Check sheet for the modelled part. Datum: model origin and axes. Units: mm. Round coordinates to 2 decimals unless told otherwise and drop trailing zeros. Write each loop counter-clockwise with the first axis right and the second up, starting at its lowest first coordinate (ties: lowest second). Pieces come first, ordered by that corner, then holes.
Item 1: Cross-section at A-A on y = 0.75. Enter the section's corners in (x, z).
Item 2: Go/stop test with flat-tipped pins: pin 1 Ø1.2 at (x, z) = (-55, -90) entering from -Y; pin 2 Ø3 at (x, z) = (55, 90) entering from +Y. Record where each tip stops, or that it passes through.
Item 3: Material ranges on line 1 (X direction, y = 0.5, z = 90); line 2 (X direction, y = 0.35, z = 68); line 3 (Z direction, x = -62, y = 1.55), recorded low to high.
Item 4: Cross-section at B-B on x = -78. Enter the section's corners in (y, z), plus the area to 3 significant figures.
from build123d import *

# Parameters (mm, degrees)
ESBO_O1_W                = 190
ESBO_O1_H                = 190
RESSALTO_EXTRUS_O1_DEPTH = 1.6
FILETE1_R                = 35
ESBO_O2_R                = 1
CORTE_EXTRUS_O1_DEPTH    = 135.359815421


with BuildPart() as part:
    # Esboço1 → Ressalto-extrusão1 (new body)
    with BuildSketch(Plane(origin=(0, 0, 0), x_dir=(1, 0, 0), z_dir=(0, 1, 0))):
        Rectangle(ESBO_O1_W, ESBO_O1_H)
    extrude(amount=RESSALTO_EXTRUS_O1_DEPTH)

    # Filete1
    filete1_edges = [part.edges().sort_by_distance(p)[0] for p in [
        (95, 0.8, 95),
        (-95, 0.8, 95),
        (-95, 0.8, -95),
        (95, 0.8, -95),
    ]]
    fillet(filete1_edges, radius=FILETE1_R)

    # Esboço2 → Corte-extrusão1 (cut, through all)
    with BuildSketch(Plane(origin=(0, 1.6, 0), x_dir=(1, 0, 0), z_dir=(0, 1, 0))):
        with Locations(Location((-55, 90, 0), (0, 0, 270))):
            Circle(ESBO_O2_R)
        with Locations(Location((55, 90, 0), (0, 0, 90))):
            Circle(ESBO_O2_R)
        with Locations(Location((55, -90, 0), (0, 0, 270))):
            Circle(ESBO_O2_R)
        with Locations(Location((-55, -90, 0), (0, 0, 90))):
            Circle(ESBO_O2_R)
    extrude(amount=-CORTE_EXTRUS_O1_DEPTH, mode=Mode.SUBTRACT)


solid = part.part
Response values:
1. outline: (-95, -60) arc R35 ccw to (-60, -95) - (60, -95) arc R35 ccw to (95, -60) - (95, 60) arc R35 ccw to (60, 95) - (-60, 95) arc R35 ccw to (-95, 60) - close; hole circle Ø2 at (-55, -90); hole circle Ø2 at (-55, 90); hole circle Ø2 at (55, -90); hole circle Ø2 at (55, 90)
2. pin 1: passes through
2. pin 2: stops at y = 1.6
3. line 1: x = -78.03 to -56, -54 to 54, 56 to 78.03
3. line 2: x = -94.07 to 94.07
3. line 3: z = -94.94 to 94.94
4. outline: (0, -90.02) - (1.6, -90.02) - (1.6, 90.02) - (0, 90.02) - close
4. area: 288 mm2
